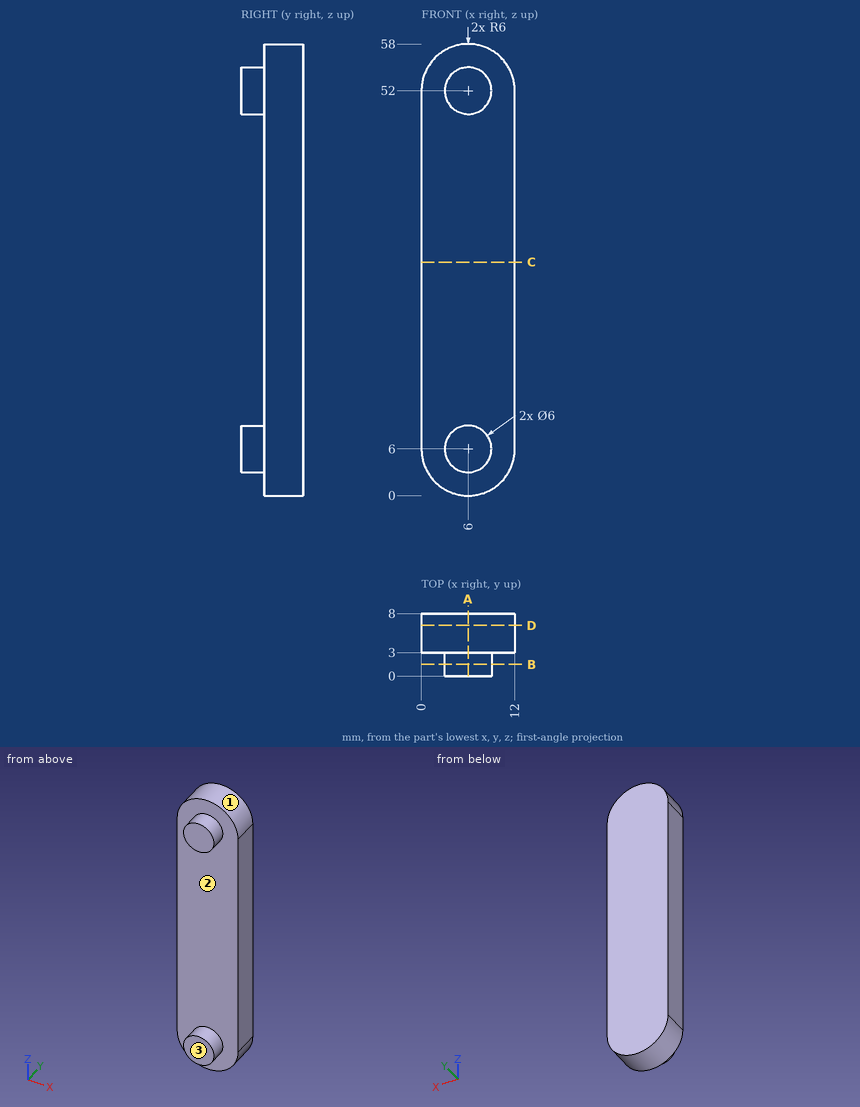
Study the drawing (mm; zero at the part's minimum x, y, z) and answer. Give positions to 0.01 mm unless a question says otherwise; leave off trailing zeros. Order: outer loops, then holes, each group sorted by start corner. A loop starts at its lowest first (then second) coordinate and runs counter-clockwise, first axis right, second up. Notation, with made-up numbers: (25, -1) - (32, -1) arc R27 cw to (32, 35) - close; hole circle Ø1 at (25.5, 11.5). An arc over 180 degrees is marked (long way). Use one line per item in the form item = value. Start each with the question number.
(1) A cutting plane is placed at B-B, the plane y = 1.5. Write down the section's boundary in (x, z).
(2) A cutting plane is placed at A-A, the plane x = 6. Write down the section's boundary in (y, z), then the cut area to 3 significant figures.
(3) Flat-ended cylindrical pins translate along their axes: pin 1 Ø6 at (x, z) = (3, 49) entering from -Y; pin 2 Ø2 at (x, y) = (8.5, 5) entering from +Z; pin 3 Ø5 at (x, z) = (9.5, 41.5) entering from -Y. Find the tip coordinate at first contact, or state that the pin passes through.
(4) A cutting plane is placed at C-C, the plane z = 30. Write down the section's boundary in (x, y), then the cut area to 3 significant figures.
(5) A cutting plane is placed at D-D, the plane y = 6.5. Write down the section's boundary in (x, z), then the cut area to 3 significant figures.
(6) Consider line 1 (Y direction, x = 8.5, z = 32.5); line 2 (Z direction, x = 6.75, y = 2); line 3 (Z direction, x = 7.25, y = 1.5). Determine where each line is inside the solid, lowest interval first. Write a range as from..to.
(7) The mould has two halves that part along Z. Classify the marked faces 1, 2 and 3: released by +Z, released by -Z, zero draft, split by the parting line, or undercut.
Ans:
q1.outline = circle Ø6 at (6, 6); circle Ø6 at (6, 52)
q2.outline = (0, 3) - (3, 3) - (3, 0) - (8, 0) - (8, 58) - (3, 58) - (3, 55) - (0, 55) - (0, 49) - (3, 49) - (3, 9) - (0, 9) - close
q2.area = 326 mm^2
q3.pin_1 = 0
q3.pin_2 = 57.81
q3.pin_3 = 3
q4.outline = (0, 3) - (12, 3) - (12, 8) - (0, 8) - close
q4.area = 60.0 mm^2
q5.outline = (0, 6) arc R6 ccw to (12, 6) - (12, 52) arc R6 ccw to (0, 52) - close
q5.area = 665 mm^2
q6.line_1 = 3..8
q6.line_2 = 3.1..8.9, 49.1..54.9
q6.line_3 = 3.27..8.73, 49.27..54.73
q7.face_1 = released by +Z
q7.face_2 = undercut
q7.face_3 = zero draft
